Autodesk Inventor part; units mm, degrees
ref_plane "YZ Plane" through (0, 0, 0) normal (1, 0, 0) x (0, 1, 0)
ref_plane "XZ Plane" through (0, 0, 0) normal (0, 1, 0) x (-1, 0, 0)
ref_plane "XY Plane" through (0, 0, 0) normal (0, 0, 1) x (1, 0, 0)
ref_plane "Arbeitsebene1" through (0, 0, 0) normal (0, 0, 1) x (1, 0, 0)
sketch "Skizze1" plane through (0, 0, 0) normal (0, 0, 1) x (1, 0, 0)
  line L0 (53.9, 111.9999) -> (53.9, 109.9999) construction
  line L1 (53.9, 109.9999) -> (-45.9, 109.9999) construction
  line L2 (-45.9, 109.9999) -> (-45.9, 111.9999) construction
  line L3 (-66.1, 111.9999) -> (-66.1, 109.9999) construction
  line L4 (-66.1, 109.9999) -> (-123.5, 109.9999) construction
  arc A0 (-123.5, 109.9999) -> (-125.5, 107.9999) centre (-123.5, 107.9999) ccw construction
  line L5 (-125.5, 107.9999) -> (-125.5, 96.9999) construction
  line L6 (-125.5, 96.9999) -> (-127.5, 96.9999) construction
  line L7 (133.5, 96.9999) -> (133.5, 107.9999) construction
  arc A1 (133.5, 107.9999) -> (131.5, 109.9999) centre (131.5, 107.9999) ccw construction
  line L8 (131.5, 109.9999) -> (74.1, 109.9999) construction
  line L9 (74.1, 109.9999) -> (74.1, 111.9999) construction
  line L10 (135.5, 96.9999) -> (133.5, 96.9999) construction
  line L11 (-45.9, -111.9999) -> (-45.9, -109.9999) construction
  line L12 (-45.9, -109.9999) -> (53.9, -109.9999) construction
  line L13 (53.9, -109.9999) -> (53.9, -111.9999) construction
  line L14 (74.1, -111.9999) -> (74.1, -109.9999) construction
  line L15 (74.1, -109.9999) -> (131.5, -109.9999) construction
  arc A2 (131.5, -109.9999) -> (133.5, -107.9999) centre (131.5, -107.9999) ccw construction
  line L16 (133.5, -107.9999) -> (133.5, -96.9999) construction
  line L17 (133.5, -96.9999) -> (135.5, -96.9999) construction
  line L18 (-125.5, -96.9999) -> (-125.5, -107.9999) construction
  arc A3 (-125.5, -107.9999) -> (-123.5, -109.9999) centre (-123.5, -107.9999) ccw construction
  line L19 (-123.5, -109.9999) -> (-66.1, -109.9999) construction
  line L20 (-66.1, -109.9999) -> (-66.1, -111.9999) construction
  line L21 (-127.5, -96.9999) -> (-125.5, -96.9999) construction
  line L22 (135.5, -96.9999) -> (135.5, 96.9999) construction
  line L23 (74.1, 111.9999) -> (53.9, 111.9999) construction
  line L24 (-45.9, 111.9999) -> (-66.1, 111.9999) construction
  line L25 (-127.5, 96.9999) -> (-127.5, -96.9999) construction
  line L26 (-127.5, -109.9999) -> (-127.5, -111.9999) construction
  line L27 (-66.1, -111.9999) -> (-45.9, -111.9999) construction
  line L28 (53.9, -111.9999) -> (74.1, -111.9999) construction
  line L29 (135.45, 96.9499) -> (133.45, 96.9499)
  line L30 (133.45, 96.9499) -> (133.45, 107.9999)
  arc A4 (133.45, 107.9999) -> (131.5, 109.9499) centre (131.5, 107.9999) ccw
  line L31 (131.5, 109.9499) -> (74.05, 109.9499)
  line L32 (74.05, 109.9499) -> (74.05, 111.9499)
  line L33 (74.05, 111.9499) -> (53.95, 111.9499)
  line L34 (53.95, 111.9499) -> (53.95, 109.9499)
  line L35 (53.95, 109.9499) -> (-45.95, 109.9499)
  line L36 (-45.95, 109.9499) -> (-45.95, 111.9499)
  line L37 (-45.95, 111.9499) -> (-66.05, 111.9499)
  line L38 (-66.05, 111.9499) -> (-66.05, 109.9499)
  line L39 (-66.05, 109.9499) -> (-123.5, 109.9499)
  arc A5 (-123.5, 109.9499) -> (-125.45, 107.9999) centre (-123.5, 107.9999) ccw
  line L40 (-125.45, 107.9999) -> (-125.45, 96.9499)
  line L41 (-125.45, 96.9499) -> (-127.45, 96.9499)
  line L42 (-127.45, 96.9499) -> (-127.45, -96.9499)
  line L43 (-127.45, -96.9499) -> (-125.45, -96.9499)
  line L44 (-125.45, -96.9499) -> (-125.45, -107.9999)
  arc A6 (-125.45, -107.9999) -> (-123.5, -109.9499) centre (-123.5, -107.9999) ccw
  line L45 (-123.5, -109.9499) -> (-66.05, -109.9499)
  line L46 (-66.05, -109.9499) -> (-66.05, -111.9499)
  line L47 (-66.05, -111.9499) -> (-45.95, -111.9499)
  line L48 (-45.95, -111.9499) -> (-45.95, -109.9499)
  line L49 (-45.95, -109.9499) -> (53.95, -109.9499)
  line L50 (53.95, -109.9499) -> (53.95, -111.9499)
  line L51 (53.95, -111.9499) -> (74.05, -111.9499)
  line L52 (74.05, -111.9499) -> (74.05, -109.9499)
  line L53 (74.05, -109.9499) -> (131.5, -109.9499)
  arc A7 (131.5, -109.9499) -> (133.45, -107.9999) centre (131.5, -107.9999) ccw
  line L54 (133.45, -107.9999) -> (133.45, -96.9499)
  line L55 (133.45, -96.9499) -> (135.45, -96.9499)
  line L56 (135.45, -96.9499) -> (135.45, 96.9499)
  circle A8 centre (99.9961, 75.0051) radius 2.25
  circle A9 centre (59.9961, 75.0041) radius 2.25
  circle A10 centre (102.9981, 0.0052) radius 2.25
  circle A11 centre (100, -74.9949) radius 2.25
  circle A12 centre (60, -74.9959) radius 2.25
  circle A13 centre (0, -74.9974) radius 2.25
  circle A14 centre (-60, -74.999) radius 2.25
  circle A15 centre (-100, -75) radius 2.25
  circle A16 centre (-100.0039, 75) radius 2.25
  circle A17 centre (-60.0039, 75.001) radius 2.25
  circle A18 centre (-0.0039, 75.0026) radius 2.25
  line L57 (100, -74.9949) -> (-100.0039, 75) construction
  line L58 (-100.0039, 75) -> (99.9961, 75.0051) construction
  line L59 (99.9961, 75.0051) -> (-100, -75) construction
  line L60 (94.9981, 68.0026) -> (-95.0019, 68.0026)
  line L61 (-95.0019, 68.0026) -> (-95.0019, -67.9974)
  line L62 (-95.0019, -67.9974) -> (94.9981, -67.9974)
  line L63 (94.9981, -67.9974) -> (94.9981, 68.0026)
  line L64 (94.9981, 68.0026) -> (-95.0019, -67.9974) construction
  line L65 (-95.0019, 68.0026) -> (94.9981, -67.9974) construction
  circle A19 centre (-103.0019, -0.0001) radius 2.25
  point P0 (0, 0)
  point P1 (-0.0019, 0.0026)
  dimension "d0" = 0.05
  dimension "d1" = 190
  dimension "d2" = 136
extrude "Grobblech1" add sketch "Skizze1" along normal blind 2
sketch "Skizze2" plane through (0, 0, 0) normal (0, 0, -1) x (-1, 0, 0)
  arc A0 (121.45, -109.9499) -> (125.45, -105.9499) centre (121.45, -105.9499) ccw
  line L0 (-94.9981, -67.9974) -> (-94.9981, 68.0026)
  line L1 (-94.9981, 68.0026) -> (95.0019, 68.0026)
  line L2 (95.0019, 68.0026) -> (95.0019, -67.9974)
  line L3 (95.0019, -67.9974) -> (-94.9981, -67.9974)
  circle A1 centre (103.0019, -0.0001) radius 2.25
  circle A2 centre (0.0039, 75.0026) radius 2.25
  circle A3 centre (60.0039, 75.001) radius 2.25
  circle A4 centre (100.0039, 75) radius 2.25
  circle A5 centre (100, -75) radius 2.25
  circle A6 centre (60, -74.999) radius 2.25
  circle A7 centre (0, -74.9974) radius 2.25
  circle A8 centre (-60, -74.9959) radius 2.25
  circle A9 centre (-100, -74.9949) radius 2.25
  circle A10 centre (-102.9981, 0.0052) radius 2.25
  circle A11 centre (-59.9961, 75.0041) radius 2.25
  circle A12 centre (-99.9961, 75.0051) radius 2.25
  line L4 (-135.45, 96.9499) -> (-133.45, 96.9499)
  line L5 (-135.45, -96.9499) -> (-135.45, 96.9499)
  line L6 (-133.45, -96.9499) -> (-135.45, -96.9499)
  line L7 (-133.45, -107.9999) -> (-133.45, -96.9499)
  arc A13 (-133.45, -107.9999) -> (-131.5, -109.9499) centre (-131.5, -107.9999) ccw
  line L8 (-74.05, -109.9499) -> (-131.5, -109.9499)
  line L9 (-74.05, -111.9499) -> (-74.05, -109.9499)
  line L10 (-53.95, -111.9499) -> (-74.05, -111.9499)
  line L11 (-53.95, -109.9499) -> (-53.95, -111.9499)
  line L12 (45.95, -109.9499) -> (-53.95, -109.9499)
  line L13 (45.95, -111.9499) -> (45.95, -109.9499)
  line L14 (66.05, -111.9499) -> (45.95, -111.9499)
  line L15 (66.05, -109.9499) -> (66.05, -111.9499)
  line L16 (123.5, -109.9499) -> (66.05, -109.9499)
  arc A14 (123.5, -109.9499) -> (125.45, -107.9999) centre (123.5, -107.9999) ccw
  line L17 (125.45, -96.9499) -> (125.45, -107.9999)
  line L18 (127.45, -96.9499) -> (125.45, -96.9499)
  line L19 (127.45, 96.9499) -> (127.45, -96.9499)
  line L20 (125.45, 96.9499) -> (127.45, 96.9499)
  line L21 (125.45, 107.9999) -> (125.45, 96.9499)
  arc A15 (125.45, 107.9999) -> (123.5, 109.9499) centre (123.5, 107.9999) ccw
  line L22 (66.05, 109.9499) -> (123.5, 109.9499)
  line L23 (66.05, 111.9499) -> (66.05, 109.9499)
  line L24 (45.95, 111.9499) -> (66.05, 111.9499)
  line L25 (45.95, 109.9499) -> (45.95, 111.9499)
  line L26 (-53.95, 109.9499) -> (45.95, 109.9499)
  line L27 (-53.95, 111.9499) -> (-53.95, 109.9499)
  line L28 (-74.05, 111.9499) -> (-53.95, 111.9499)
  line L29 (-74.05, 109.9499) -> (-74.05, 111.9499)
  line L30 (-131.5, 109.9499) -> (-74.05, 109.9499)
  arc A16 (-131.5, 109.9499) -> (-133.45, 107.9999) centre (-131.5, 107.9999) ccw
  line L31 (-133.45, 96.9499) -> (-133.45, 107.9999)
  arc A17 (125.45, 105.9499) -> (121.45, 109.9499) centre (121.45, 105.9499) ccw
  arc A18 (-129.45, 109.9499) -> (-133.45, 105.9499) centre (-129.45, 105.9499) ccw
  line L32 (-133.45, 96.9499) -> (-133.45, 107.9999)
  arc A19 (-133.45, -105.9499) -> (-129.45, -109.9499) centre (-129.45, -105.9499) ccw
  line L33 (-133.45, -107.9999) -> (-133.45, -96.9499)
  line L34 (-74.05, -109.9499) -> (-131.5, -109.9499)
  point P0 (0, 0)
  dimension "d4" = 8
  dimension "d5" = 8
  dimension "d6" = 8
  dimension "d7" = 8
extrude "Extrusion1" cut sketch "Skizze2" against normal through all contours A0 L17 A14 L16 | A17 L22 A15 L21 | L8 A13 L7 A19 | L31 A16 L30 A18
equation "\"d3\" = Stärke"
equation "\"Biegeradius\" = Stärke"
equation "\"BreiteBiegungsfreistellung\" = Stärke"
equation "\"TiefeBiegungsfreistellung\" = 0.5 * Stärke"
equation "\"GrößeEckenfreistellung\" = 4 * Stärke"
equation "\"MinimalRest\" = 2 * Stärke"
equation "\"Übergangsradius\" = Biegeradius"
equation "\"JacobiRadiusGröße\" = Biegeradius"
equation "\"Abstandsgröße\" = Stärke"
properties part number "BrennerHalter"
Source: CAD feature listing. Evaluate the final solid. Frame: model axes, mm. Give positions to 0.01 mm unless a question says otherwise; leave off trailing zeros. Order: outer loops, then holes, each group sorted by start corner. A loop starts at its lowest first (then second) coordinate and runs counter-clockwise, first axis right, second up. Notation, with made-up numbers: (-9, 12.25) -> (46, 12.25) arc R8 cw to (46, 19.25) -> close; hole circle Ø4 at (5, 47). An arc over 180 degrees is marked (long way). Use a Markdown table: item, result.
Q1. Section B-B (x = 116.5). Return the cut outline in (y, z), and give its area (3 significant figures).
A:
| item | result |
|---|---|
| outline | (-109.95, 0) -> (109.95, 0) -> (109.95, 2) -> (-109.95, 2) -> close |
| area | 440 mm^2 |
Q2. First-contact query: P1, Ø1, axis at x = 135, z = 1.5, coming from the +Y side; P2, Ø1, axis at y = 100.5, z = 0.5, coming from the +X side; P3, Ø3.5, axis at x = -60, y = -74.999, coming from the +Z side; P4, Ø0.6, axis at y = -110.5, z = 1, coming from the -X side. Flat tips, straight axial feed; report the tip coordinate or a pass-through.
A:
| item | result |
|---|---|
| P1 | y = 96.95 |
| P2 | x = 133.45 |
| P3 | through |
| P4 | x = -66.05 |
Q3. Section A-A (y = -40). Return the cut outline in (x, z), and give its area (3 significant figures).
A:
| item | result |
|---|---|
| outline | (-127.45, 0) -> (-95, 0) -> (-95, 2) -> (-127.45, 2) -> close; (95, 0) -> (135.45, 0) -> (135.45, 2) -> (95, 2) -> close |
| area | 146 mm^2 |
Q4. Material intervals for line 1 (Y direction, x = 0, z = 0.85); line 2 (Y direction, x = 100, z = 1.35); line 3 (Y direction, x = -86.5, z = 1.35), sorted ascending. Write a range as [from, to].
A:
| item | result |
|---|---|
| line 1 | [-109.95, -77.25], [-72.75, -68], [68, 72.75], [77.25, 109.95] |
| line 2 | [-109.95, -77.24], [-72.74, 72.76], [77.26, 109.95] |
| line 3 | [-109.95, -68], [68, 109.95] |
Q5. Section C-C (z = 1.7). State how many separate pieces and enclosed holes the cut face has, and give its area (3 significant figures).
A:
| item | result |
|---|---|
| separate pieces | 1 |
| enclosed holes | 13 |
| area | 31,800 mm^2 |
